Geometry check sheet. Reference: the model listing, model coordinates, mm. A direction names the side the tool comes from. Round coordinates to 2 decimals unless told otherwise and drop trailing zeros.
```python
from build123d import *

# Parameters (mm, degrees)
F0_R      = 6.25
F1_DEPTH  = 13
F0_R_2    = 4.75
F0_R_3    = 4
F2_DEPTH  = 2
F3_DEPTH  = 8.6
F4_R      = 1
F5_R      = 4
F7_DEPTH  = 6.4553484435
F5_R_2    = 1
F8_DEPTH  = 2
F6_R      = 4
F9_DEPTH  = 6.4553484442
F6_R_2    = 1
F10_DEPTH = 2
F11_DEPTH = 1
F12_R     = 1
F13_DEPTH = 2


with BuildPart() as f1:
    # F0 (on Front) → F1 (new body)
    with BuildSketch(Plane.XZ):
        with BuildLine():
            Line((-11, -4.5), (-11, -7.5))
            Line((-11, -7.5), (11, -7.5))
            Line((11, -7.5), (11, -4.5))
            Line((11, -4.5), (10, -4.5))
            ThreePointArc((10, -4.5), (8.2641129984, -3.493325887), (8.2756985044, -1.4866963178))
            Line((8.2756985044, -1.4866963178), (11, 3.1491470389))
            Line((11, 3.1491470389), (0, 9.5))
            Line((0, 9.5), (-11, 3.1491470389))
            Line((-11, 3.1491470389), (-8.2756985044, -1.4866963178))
            ThreePointArc((-8.2756985044, -1.4866963178), (-8.2641129984, -3.493325887), (-10, -4.5))
            Line((-10, -4.5), (-11, -4.5))
        make_face()
        Circle(F0_R, mode=Mode.SUBTRACT)
    extrude(amount=F1_DEPTH)

    # F0 (on Front) → F2 (join)
    with BuildSketch(Plane.XZ):
        with BuildLine():
            Line((-11, -4.5), (-11, -7.5))
            Line((-11, -7.5), (11, -7.5))
            Line((11, -7.5), (11, -4.5))
            Line((11, -4.5), (10, -4.5))
            ThreePointArc((10, -4.5), (8.2641129984, -3.493325887), (8.2756985044, -1.4866963178))
            Line((8.2756985044, -1.4866963178), (11, 3.1491470389))
            Line((11, 3.1491470389), (0, 9.5))
            Line((0, 9.5), (-11, 3.1491470389))
            Line((-11, 3.1491470389), (-8.2756985044, -1.4866963178))
            ThreePointArc((-8.2756985044, -1.4866963178), (-8.2641129984, -3.493325887), (-10, -4.5))
            Line((-10, -4.5), (-11, -4.5))
        make_face()
        Circle(F0_R, mode=Mode.SUBTRACT)
        Circle(F0_R)
        Circle(F0_R_2, mode=Mode.SUBTRACT)
        Circle(F0_R_2)
        Circle(F0_R_3, mode=Mode.SUBTRACT)
    extrude(amount=-F2_DEPTH)

    # F0 (on Front) → F3 (join)
    with BuildSketch(Plane.XZ):
        Circle(F0_R_2)
        Circle(F0_R_3, mode=Mode.SUBTRACT)
    extrude(amount=-F3_DEPTH)

    # F4
    f4_edges = [f1.edges().sort_by_distance(p)[0] for p in [
        (-4.75, 2, 0),
    ]]
    fillet(f4_edges, radius=F4_R)

    # F5 (on face) → F7 (cut, up to face)
    with BuildSketch(Plane(origin=(4.113620668, 0, 7.125), x_dir=(0.8660254038, 0, -0.5), z_dir=(0.5, 0, 0.8660254038))):
        with Locations((1.6017059222, -6.5)):
            Circle(F5_R)
    extrude(amount=-F7_DEPTH, mode=Mode.SUBTRACT)

    # F5 (on face) → F8 (cut)
    with BuildSketch(Plane(origin=(4.113620668, 0, 7.125), x_dir=(0.8660254038, 0, -0.5), z_dir=(0.5, 0, 0.8660254038))):
        with Locations((-2.8982940778, -2)):
            Circle(F5_R_2)
        with Locations((6.1017059222, -2)):
            Circle(F5_R_2)
        with Locations((6.1017059222, -11)):
            Circle(F5_R_2)
        with Locations((-2.8982940778, -11)):
            Circle(F5_R_2)
    extrude(amount=-F8_DEPTH, mode=Mode.SUBTRACT)

    # F6 (on face) → F9 (cut, up to face)
    with BuildSketch(Plane(origin=(-4.113620668, 0, 7.125), x_dir=(0.8660254038, 0, 0.5), z_dir=(-0.5, 0, 0.8660254038))):
        with Locations((-1.6017059222, -4.5)):
            Circle(F6_R)
    extrude(amount=-F9_DEPTH, mode=Mode.SUBTRACT)

    # F6 (on face) → F10 (cut)
    with BuildSketch(Plane(origin=(-4.113620668, 0, 7.125), x_dir=(0.8660254038, 0, 0.5), z_dir=(-0.5, 0, 0.8660254038))):
        with Locations((-6.1017059222, -9)):
            Circle(F6_R_2)
        with Locations((-6.1017059222, 0)):
            Circle(F6_R_2)
        with Locations((2.8982940778, 0)):
            Circle(F6_R_2)
        with Locations((2.8982940778, -9)):
            Circle(F6_R_2)
    extrude(amount=-F10_DEPTH, mode=Mode.SUBTRACT)

    # F0 (on Front) → F11 (cut)
    with BuildSketch(Plane.XZ):
        Circle(F0_R)
        Circle(F0_R_2, mode=Mode.SUBTRACT)
        Circle(F0_R_2)
        Circle(F0_R_3, mode=Mode.SUBTRACT)
    extrude(amount=-F11_DEPTH, mode=Mode.SUBTRACT)

    # F12 (on face) → F13 (cut)
    with BuildSketch(Plane(origin=(0, 0, -7.5), x_dir=(1, 0, 0), z_dir=(0, 0, -1))):
        with Locations((-6, 5.5)):
            Circle(F12_R)
        with Locations((6, 5.5)):
            Circle(F12_R)
    extrude(amount=-F13_DEPTH, mode=Mode.SUBTRACT)


solid = f1.part
```
(1) Draft check along Y on faces 5 (the flat face through (-6, -6, -5.5)), 6 (the flat face through (0.59, -1.99, 6.85)), 7 (the flat face through (9.62, -5.6, 0.8)), 8 (the flat face through (1.3, 1, -4.1)). Enter one of: released by +Y, released by -Y, zero draft, split by the parting line, or undercut.
Returned:
face 5: undercut
face 6: undercut
face 7: zero draft
face 8: released by -Y
(2) Set-up check for faces 1 (the flat face through (-10.5, -5.6, -4.5)), 2 (the cylindrical face through (5.263, -6.176, -6.514)), 3 (the flat face through (-11, -6, -6)), 4 (the flat face through (0.59, -10.99, 6.85)): record each of +Z, -Z, +X, -X, +Y, -Y from which the full face is reachable in a straight line by a thin tool's end or side.
Returned:
face 1: -X, +Y, -Y
face 2: -Z
face 3: +Z, -Z, -X, +Y, -Y
face 4: none
(3) Material ranges on line 1 (X direction, y = -5.5, z = -7.1); line 2 (Y direction, x = 6, z = -6.4); line 3 (Z direction, x = 0, y = 4), recorded low to high.
Returned:
line 1: x = -11 to -7, -5 to 5, 7 to 11
line 2: y = -13 to -6.5, -4.5 to 2
line 3: z = -4.75 to -4, 4 to 4.75
(4) Depth check by flat-ended pin: P1, Ø2.5, axis at x = 6, y = -5.5, coming from the +Z side; P2, Ø12, axis at x = -7.5, y = -5.5, coming from the +Z side; P3, Ø10, axis at x = 3, z = 1, coming from the -Y side; P4, Ø0.8, axis at x = -10.5, y = -6.5, coming from the +Z side. Enter the tip coordinate at first touch or a pass-through.
Returned:
P1: stops at z = 1.76
P2: stops at z = 8.63
P3: stops at y = -13
P4: stops at z = 3.67
